Source: CAD feature listing. Evaluate the final solid. Frame: model axes, mm. A direction names the side the tool comes from. Give positions to 0.01 mm unless a question says otherwise; leave off trailing zeros. Order: outer loops, then holes, each group sorted by start corner. A loop starts at its lowest first (then second) coordinate and runs counter-clockwise, first axis right, second up.
1) Section B-B, the plane z = 9.5. Return loops of the section in (x, y).
2) Section A-A, the plane x = 41.5. Return loops of the section in (y, z) (3 decimals), plus the area to 3 significant figures.
3) Draft query along X for faces 6 (the face through (127, -31, -25)), 7 (the face through (115, -40, 57.15)), 8 (the face through (-91.44, -40, 67)). Return one class per face: released by +X, released by -X, zero draft, split by the parting line, or undercut.
4) Material intervals for line 1 (Y direction, x = -19, z = 57); line 2 (Z direction, x = 68.5, y = -44.5); line 3 (Y direction, x = -106, z = 5.5), sorted ascending.
5) Access query for faces 1 (the face through (104.14, -40, 67)), 2 (the face through (-2, -50.8, 1)), 3 (the face through (-1, -40, 57.15)), 4 (the face through (-104.14, -40, 67)), 5 (the face through (98, -42, 76.2)). Directions: +Z, -Z, +X, -X, +Y, -Y. A direction counts if a zero-diameter tool reaches every point of the face in a straight line with its end or side. Return the directions, or none.
6) First-contact query: P1, Ø17.5, axis at x = -27.5, y = -37, coming from the +Z side; P2, Ø24, axis at x = 117.5, y = -42, coming from the +Z side; P3, Ø10, axis at x = -29.5, z = -22, coming from the +Y side. Flat tips, straight axial feed; report the tip coordinate or a pass-through.
```python
from build123d import *

# Parameters (mm, degrees)
F0_W     = 254
F0_H     = 152.4
F1_DEPTH = 50.8
F3_DEPTH = 254.001
F4_W     = 22.86
F4_H     = 19.05
F4_W_2   = 182.88
F5_DEPTH = 50.801


with BuildPart() as f1:
    # F0 (on Front) → F1 (new body)
    with BuildSketch(Plane.XZ):
        Rectangle(F0_W, F0_H)
    extrude(amount=F1_DEPTH)

    # F2 (on face) → F3 (cut, through all)
    with BuildSketch(Plane.YZ.offset(127)):
        Polygon((-33.228574, 76.2), (0, -76.2), (0, 76.2), align=None)
    extrude(amount=-F3_DEPTH, mode=Mode.SUBTRACT)

    # F4 (on face) → F5 (cut, through all)
    with BuildSketch(Plane.XZ.offset(50.8)):
        with Locations((-115.57, 66.675)):
            Rectangle(F4_W, F4_H)
        with Locations((0, 66.675)):
            Rectangle(F4_W_2, F4_H)
        with Locations((115.57, 66.675)):
            Rectangle(F4_W, F4_H)
    extrude(amount=-F5_DEPTH, mode=Mode.SUBTRACT)


solid = f1.part
```
From the geometry:
1. outline: (-127, -50.8) - (127, -50.8) - (127, -18.69) - (-127, -18.69) - close
2. outline: (-50.8, -76.2) - (0, -76.2) - (-29.075, 57.15) - (-50.8, 57.15) - close
2. area: 4,840 mm2
3. face 6: released by +X
3. face 7: zero draft
3. face 8: undercut
4. line 1: y = -50.8 to -29.04
4. line 2: z = -76.2 to 57.15
4. line 3: y = -50.8 to -17.81
5. face 1: +Z, +X, +Y, -Y
5. face 2: +Z, -Z, +X, -X, -Y
5. face 3: +Z, +Y, -Y
5. face 4: +Z, -X, +Y, -Y
5. face 5: +Z, +X, -X, +Y, -Y
6. P1: stops at z = 57.15
6. P2: stops at z = 57.15
6. P3: stops at y = -10.73
